```python
from build123d import *

# Parameters (mm, degrees)
EXTRUDE086_DEPTH = 0.8
EXTRUDE087_DEPTH = 2
SKETCH084_R      = 1.8
EXTRUDE084_DEPTH = 1.6
SKETCH082_W      = 82.8
SKETCH082_H      = 36
SKETCH082_R      = 1.8
EXTRUDE082_DEPTH = 1.6
SKETCH076_R      = 7.3
EXTRUDE077_DEPTH = 1.2
SKETCH074_R      = 1.8
SKETCH074_R_2    = 6.3
EXTRUDE076_DEPTH = 2


with BuildPart() as obj1:
    # Sketch086 → Extrude086 (new body)
    with BuildSketch(Plane(origin=(0, 0, 2), x_dir=(1, 0, 0), z_dir=(0, -1, 0))):
        with BuildLine():
            Line((-137.814627, 37.2), (-144.028897, 18.074442))
            ThreePointArc((-132.428405, 21.823197), (-138.523989, 20.862741), (-144.028897, 18.074442))
            Line((-120.896651, 21.823197), (-132.428405, 21.823197))
            ThreePointArc((-120.896651, 21.823197), (-116.782154, 23.160078), (-114.239255, 26.660078))
            Line((-110.814627, 37.2), (-114.239255, 26.660078))
            Line((-137.814627, 37.2), (-110.814627, 37.2))
        make_face()
    extrude(amount=-EXTRUDE086_DEPTH)


with BuildPart() as obj1_1:
    # Extrude086 placement: moved
    add(obj1.part.moved(Location((0, 2, 0))))


with BuildPart() as extrude087:
    # Sketch087 → Extrude087 (new body)
    with BuildSketch(Plane.XZ):
        with BuildLine():
            add(Edge.make_bspline(
                [(-183.167024, 31.421083), (-188.478801, 29.986374), (-187.676319, 25.030408), (-186.873836, 20.074442), (-181.329747, 20.074442)],
                knots=[5.002901, 5.002901, 5.002901, 6.428441, 6.428441, 7.853982, 7.853982, 7.853982], degree=2, weights=[1, 0.756553, 1, 0.756553, 1]))
            Line((-181.329747, 20.074442), (-144.028897, 20.074442))
            Line((-144.028897, 20.074442), (-137.814627, 39.2))
            Line((-137.814627, 39.2), (-178.753577, 39.2))
            Line((-178.753577, 39.2), (-180.790744, 33.602929))
            ThreePointArc((-180.790744, 33.602929), (-181.712516, 32.221901), (-183.167024, 31.421083))
        make_face()
    extrude(amount=-EXTRUDE087_DEPTH)


with BuildPart() as extrude087_1:
    # Extrude087 placement: moved
    add(extrude087.part.moved(Location((0, 2, 0))))


with BuildPart() as extrude084:
    # Sketch084 → Extrude084 (new body)
    with BuildSketch(Plane.XZ):
        with BuildLine():
            ThreePointArc((-78.51, 31.3), (-76.035126, 32.325126), (-75.01, 34.8))
            Line((-75.01, 39.2), (-75.01, 34.8))
            Line((-82.8, 39.2), (-75.01, 39.2))
            Line((-82.8, 31.3), (-82.8, 39.2))
            Line((-82.8, 31.3), (-78.51, 31.3))
        make_face()
        with Locations((-78.51, 34.8)):
            Circle(SKETCH084_R, mode=Mode.SUBTRACT)
        with BuildLine():
            ThreePointArc((-9.1, 34.8), (-8.074874, 32.325126), (-5.6, 31.3))
            Line((-5.6, 31.3), (0, 31.3))
            Line((0, 39.2), (0, 31.3))
            Line((-9.1, 39.2), (0, 39.2))
            Line((-9.1, 39.2), (-9.1, 34.8))
        make_face()
        with Locations((-5.6, 34.8)):
            Circle(SKETCH084_R, mode=Mode.SUBTRACT)
        with BuildLine():
            ThreePointArc((-75.01, 7.6), (-76.035126, 10.074874), (-78.51, 11.1))
            Line((-82.8, 11.1), (-78.51, 11.1))
            Line((-82.8, 3.2), (-82.8, 11.1))
            Line((-75.01, 3.2), (-82.8, 3.2))
            Line((-75.01, 7.6), (-75.01, 3.2))
        make_face()
        with Locations((-78.51, 7.6)):
            Circle(SKETCH084_R, mode=Mode.SUBTRACT)
        with BuildLine():
            ThreePointArc((-5.6, 11.1), (-8.074874, 10.074874), (-9.1, 7.6))
            Line((-9.1, 7.6), (-9.1, 3.2))
            Line((0, 3.2), (-9.1, 3.2))
            Line((0, 11.1), (0, 3.2))
            Line((0, 11.1), (-5.6, 11.1))
        make_face()
        with Locations((-5.6, 7.6)):
            Circle(SKETCH084_R, mode=Mode.SUBTRACT)
    extrude(amount=-EXTRUDE084_DEPTH)


with BuildPart() as extrude084_1:
    # Extrude084 placement: moved
    add(extrude084.part.moved(Location((0, 2, 0))))


with BuildPart() as cut047:
    # Sketch082 → Extrude082 (new body)
    with BuildSketch(Plane.XZ):
        with Locations((-41.4, 21.2)):
            Rectangle(SKETCH082_W, SKETCH082_H)
        with Locations((-78.51, 34.8)):
            Circle(SKETCH082_R, mode=Mode.SUBTRACT)
        with Locations((-5.6, 34.8)):
            Circle(SKETCH082_R, mode=Mode.SUBTRACT)
        with Locations((-5.6, 7.6)):
            Circle(SKETCH082_R, mode=Mode.SUBTRACT)
        with Locations((-78.51, 7.6)):
            Circle(SKETCH082_R, mode=Mode.SUBTRACT)
        with BuildLine():
            ThreePointArc((-65, 31.2), (-75, 21.2), (-65, 11.2))
            Line((-65, 11.2), (-19, 11.2))
            ThreePointArc((-19, 11.2), (-9, 21.2), (-19, 31.2))
            Line((-65, 31.2), (-19, 31.2))
        make_face(mode=Mode.SUBTRACT)
    extrude(amount=-EXTRUDE082_DEPTH)


with BuildPart() as cut047_1:
    # Extrude082 placement: moved
    add(cut047.part.moved(Location((0, 2, 0))))

    # Cut047: cut Extrude084
    add(extrude084_1.part, mode=Mode.SUBTRACT)


with BuildPart() as obj2:
    # Sketch076 → Extrude077 (new body)
    with BuildSketch(Plane.XZ):
        with Locations((-65, 21.2)):
            Circle(SKETCH076_R)
        with Locations((-42, 21.2)):
            Circle(SKETCH076_R)
        with Locations((-19, 21.2)):
            Circle(SKETCH076_R)
    extrude(amount=-EXTRUDE077_DEPTH)


with BuildPart() as fusion007:
    # Sketch074 → Extrude076 (new body)
    with BuildSketch(Plane.XZ):
        with BuildLine():
            Line((-82.8, 3.2), (0, 3.2))
            Line((0, 3.2), (0, 39.2))
            Line((-195.886839, 39.2), (0, 39.2))
            Line((-202.764796, 20.302968), (-195.886839, 39.2))
            ThreePointArc((-192.175575, -3.18451), (-192.085048, 10.987093), (-202.764796, 20.302968))
            Line((-192.175575, -3.18451), (-215.419579, -53.031439))
            ThreePointArc((-215.419579, -53.031439), (-218.578907, -66.677212), (-215.93199, -80.431568))
            Line((-215.93199, -80.431568), (-176.68528, -80.431568))
            Line((-147.645309, 8.944272), (-176.68528, -80.431568))
            ThreePointArc((-132.428405, 20), (-141.832969, 16.944272), (-147.645309, 8.944272))
            Line((-132.428405, 20), (-107.6, 20))
            ThreePointArc((-91.751972, 6.2), (-97.09286, 16.066483), (-107.6, 20))
            Line((-82.8, 6.2), (-91.751972, 6.2))
            Line((-82.8, 3.2), (-82.8, 6.2))
        make_face()
        with Locations((-213.443268, -76.831568)):
            Circle(SKETCH074_R, mode=Mode.SUBTRACT)
        with Locations((-179.304663, -76.831568)):
            Circle(SKETCH074_R, mode=Mode.SUBTRACT)
        with Locations((-184.079668, 34.8)):
            Circle(SKETCH074_R, mode=Mode.SUBTRACT)
        with Locations((-78.51, 34.8)):
            Circle(SKETCH074_R, mode=Mode.SUBTRACT)
        with Locations((-78.51, 7.6)):
            Circle(SKETCH074_R, mode=Mode.SUBTRACT)
        with Locations((-5.6, 34.8)):
            Circle(SKETCH074_R, mode=Mode.SUBTRACT)
        with Locations((-5.6, 7.6)):
            Circle(SKETCH074_R, mode=Mode.SUBTRACT)
        with Locations((-19, 21.2)):
            Circle(SKETCH074_R_2, mode=Mode.SUBTRACT)
        with Locations((-42, 21.2)):
            Circle(SKETCH074_R_2, mode=Mode.SUBTRACT)
        with Locations((-65, 21.2)):
            Circle(SKETCH074_R_2, mode=Mode.SUBTRACT)
        Polygon((-189.938695, 31.567195), (-192.332836, 24.989347), (-196.467483, 26.494236), (-194.073342, 33.072084), (-193.885404, 33.00368), (-190.126633, 31.635599), align=None, mode=Mode.SUBTRACT)
    extrude(amount=-EXTRUDE076_DEPTH)

    # Cut044: cut obj2
    add(obj2.part, mode=Mode.SUBTRACT)

    # Fusion005: union Cut047
    add(cut047_1.part)

    # Fusion007: union obj1, Extrude087
    add(obj1_1.part)
    add(extrude087_1.part)


solid = fusion007.part
```
Input: part model. Units: mm. Frame: model coordinates. A direction names the side the tool comes from. Round coordinates to 2 decimals unless told otherwise and drop trailing zeros. Loops run counter-clockwise (first coordinate to the right, second up) from the corner with the lowest first, then second, coordinate; pieces in that order, holes last.
1) Material intervals for line 1 (Z direction, x = -65, y = 0.95); line 2 (Z direction, x = -5.6, y = 1.55); line 3 (Y direction, x = -166, z = -3), sorted ascending.
Ans:
line 1: z = 3.2 to 13.9, 28.5 to 39.2
line 2: z = 3.2 to 5.8, 9.4 to 33, 36.6 to 39.2
line 3: y = 0 to 2
2) Section query A-A on x = -42. Return the cut outline in (y, z).
Ans:
outline: (0, 3.2) - (3.6, 3.2) - (3.6, 11.2) - (2, 11.2) - (2, 14.9) - (1.2, 14.9) - (1.2, 13.9) - (0, 13.9) - close; (0, 28.5) - (1.2, 28.5) - (1.2, 27.5) - (2, 27.5) - (2, 31.2) - (3.6, 31.2) - (3.6, 39.2) - (0, 39.2) - close
3) Section query C-C on x = -101.5. Return the cut outline in (y, z).
Ans:
outline: (0, 18.79) - (2, 18.79) - (2, 39.2) - (0, 39.2) - close
4) Pull-direction query (Z, two-part tool) for faces 1 (the flat face through (-203.635, 0.986, -27.759)), 2 (the flat face through (-161.962, 0.986, -35.118)), 3 (the cylindrical face through (-49.293, 0.592, 21.521)), 4 (the flat face through (-150, 0, 6)); classes: released by +Z, released by -Z, zero draft, split by the parting line, or undercut.
Ans:
face 1: undercut
face 2: released by -Z
face 3: undercut
face 4: zero draft
5) Pin query (flat end, axial travel): pin 1 (0.8 mm diameter, centred on y = 3, z = 4.5, fed in from -X); pin 2 (7.5 mm diameter, centred on x = -19.5, z = 24, fed in from -Y); pin 3 (0.8 mm diameter, centred on x = -2.5, y = 3, fed in from -Z). Return the tip coordinate at first contact, or that it passes through.
Ans:
pin 1: stops at x = -75.01
pin 2: stops at y = 1.2
pin 3: stops at z = 11.1
6) Set-up query: faces 5 (the cylindrical face through (-141.719, 0.986, 17.026)), 6 (the cylindrical face through (-116.832, 2.394, 25.124)), 7 (the cylindrical face through (-72.293, 0.592, 21.521)), 8 (the flat face through (-42, 3.6, 9)), 9 (the cylindrical face through (-9, 3, 21)). Return all of +Z, -Z, +X, -X, +Y, -Y with unobstructed straight access to the full face (end or side cutting, diameter ignored); none if empty.
Ans:
face 5: -Z, +Y, -Y
face 6: -Z, +Y
face 7: -Y
face 8: +Z, -Z, +X, +Y
face 9: +Y
7) Section query B-B on z = -72. Return the cut outline in (x, y).
Ans:
outline: (-218.26, 0) - (-173.95, 0) - (-173.95, 2) - (-218.26, 2) - close
